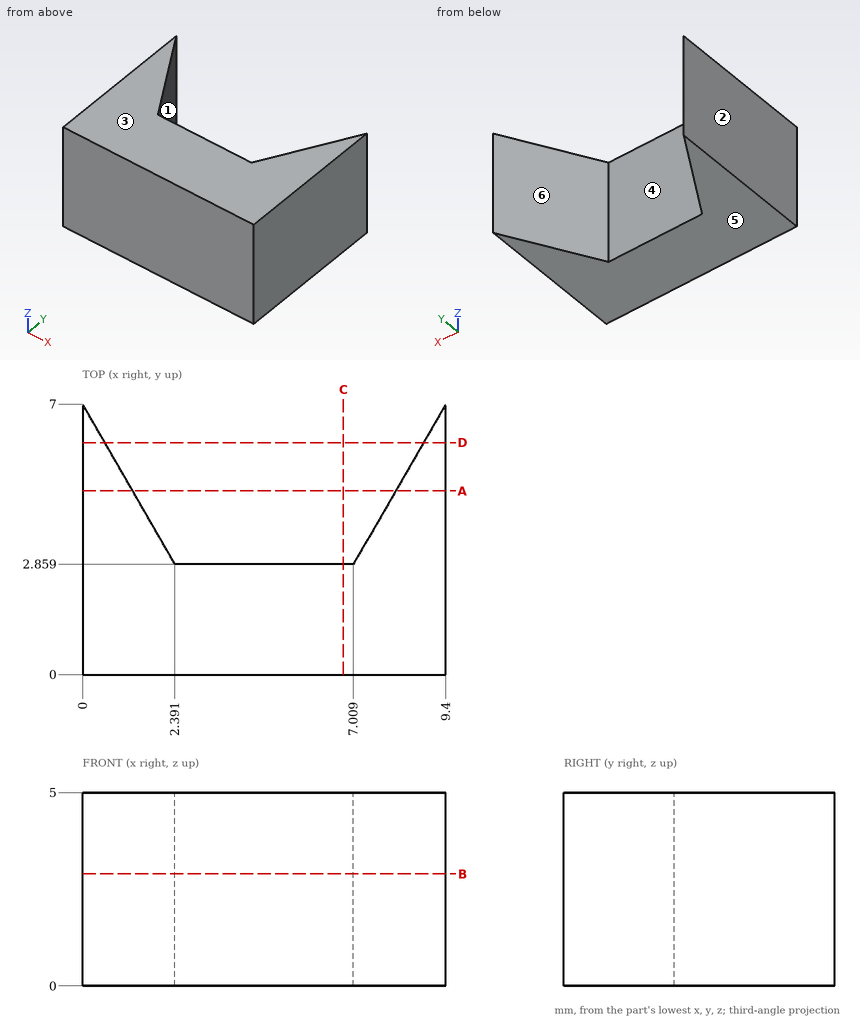
Study the drawing (mm; zero at the part's minimum x, y, z) and answer. A direction names the side the tool comes from. Give positions to 0.01 mm unless a question says otherwise; leave off trailing zeros. Order: outer loops, then holes, each group sorted by start corner. A loop starts at its lowest first (then second) coordinate and runs counter-clockwise, first axis right, second up. Notation, with made-up numbers: (77.5, 77.5) - (127.5, 77.5) arc R19 cw to (127.5, 92.5) - close; hole circle Ø5 at (20.5, 76). An arc over 180 degrees is marked (long way). Answer as CSV lines item,"result". Start each with the question number.
Q1. The mould has two halves that part along X. Classify the marked faces 1, 2, 3 and 4: +X half, -X half, draft (parallel to the pull), parting line (faces both ways), or undercut.
Q2. The part is cut by section C-C (x = 6.75). Write down the section's boundary in (y, z), then the cut area to 3 significant figures.
Q3. For the marked faces 5 and 6, determine the directions among +Z, -Z, +X, -X, +Y, -Y from which every point of the face is accessible in a straight line to the end or side of a thin tool.
Q4. Given pin 1 Ø1 at (x, z) = (1.5, 1.5) entering from +Y, flat-ended and moving along its own axis, determine where the tip first touches the part or whether it passes through.
Q5. The part is cut by section A-A (y = 4.75). Write down the section's boundary in (x, z).
Q6. Find the intervals of material crossed by L1, parallel to Y at x = 4.25, z = 0.4; L2, parallel to X at y = 5.75, z = 4.1; L3, parallel to X at y = 3.75, z = 2.6 (1 decimal), in increasing order. Write a range as [from, to].
Q7. The part is cut by section B-B (z = 2.9). Write down the section's boundary in (x, y).
Q8. The part is cut by section D-D (y = 6). Write down the section's boundary in (x, z).
Check result:
1,face 1,"undercut"
1,face 2,"-X half"
1,face 3,"draft"
1,face 4,"undercut"
2,outline,"(0, 0) - (2.86, 0) - (2.86, 5) - (0, 5) - close"
2,area,"14.3 mm²"
3,face 5,"-Z, +X, -X, +Y, -Y"
3,face 6,"+Z, -Z, +Y"
4,pin 1,"stops at y = 5.27"
5,outline,"(0, 0) - (1.3, 0) - (1.3, 5) - (0, 5) - close; (8.1, 0) - (9.4, 0) - (9.4, 5) - (8.1, 5) - close"
6,L1,"y = [0, 2.86]"
6,L2,"x = [0, 0.72], [8.68, 9.4]"
6,L3,"x = [0, 1.9], [7.5, 9.4]"
7,outline,"(0, 0) - (9.4, 0) - (9.4, 7) - (7.01, 2.86) - (2.39, 2.86) - (0, 7) - close"
8,outline,"(0, 0) - (0.58, 0) - (0.58, 5) - (0, 5) - close; (8.82, 0) - (9.4, 0) - (9.4, 5) - (8.82, 5) - close"
